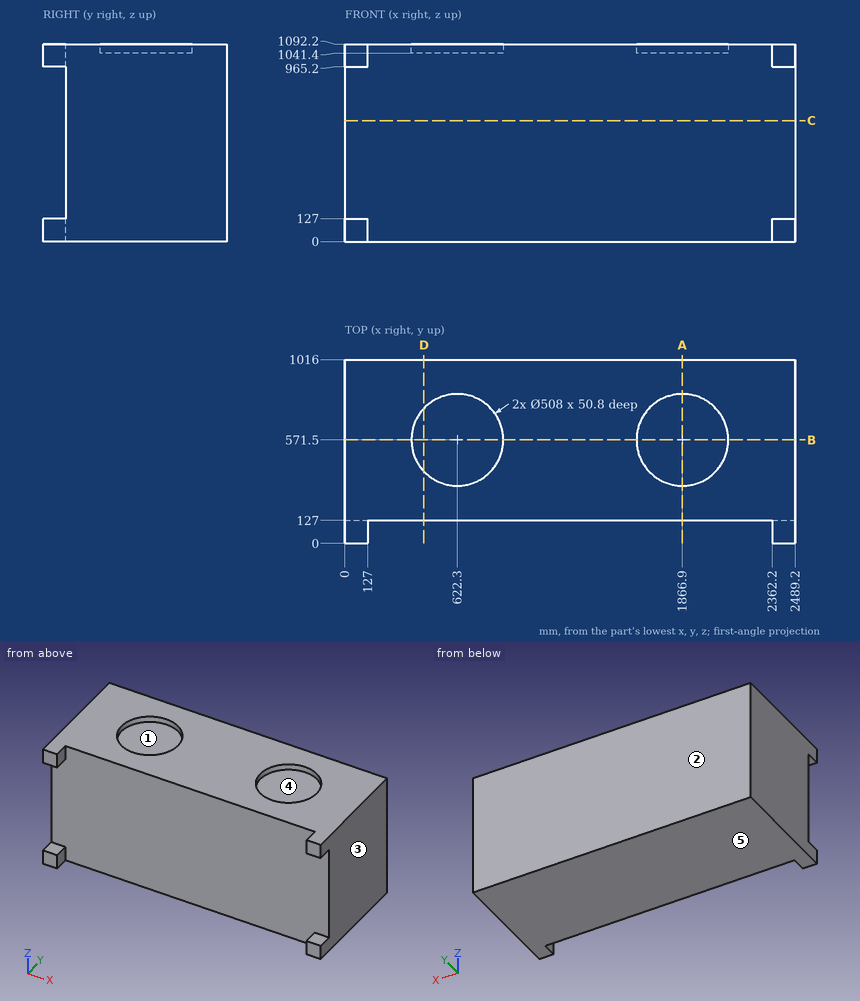
Design review of the part shown in the three views and the two pictorial views. Dimensions are in mm from the part's minimum x, y and z. A direction names the side the tool comes from. Round coordinates to 2 decimals unless told otherwise and drop trailing zeros. Order: outer loops, then holes, each group sorted by start corner. A loop starts at its lowest first (then second) coordinate and runs counter-clockwise, first axis right, second up.
(1) Take a section at B-B, the plane y = 571.5. State the section outline as (x, z) points, plus the area to 3 significant figures.
Working result:
outline: (0, 0) - (2489.2, 0) - (2489.2, 1092.2) - (2120.9, 1092.2) - (2120.9, 1041.4) - (1612.9, 1041.4) - (1612.9, 1092.2) - (876.3, 1092.2) - (876.3, 1041.4) - (368.3, 1041.4) - (368.3, 1092.2) - (0, 1092.2) - close
area: 2,670,000 mm2
(2) Take a section at C-C, the plane z = 668.5. State the section outline as (x, y) points, plus the area to 3 significant figures.
Working result:
outline: (0, 127) - (2489.2, 127) - (2489.2, 1016) - (0, 1016) - close
area: 2,210,000 mm2
(3) Take a section at A-A, the plane x = 1866.9. State the section outline as (y, z) points, plus the area to 3 significant figures.
Working result:
outline: (127, 0) - (1016, 0) - (1016, 1092.2) - (825.5, 1092.2) - (825.5, 1041.4) - (317.5, 1041.4) - (317.5, 1092.2) - (127, 1092.2) - close
area: 945,000 mm2
(4) For P1, Ø1, axis at x = 1114.5, z = 912.5, coming from the -Y side; P2, Ø3, axis at x = 1753.5, y = 791.5, coming from the +Z side, all flat-tipped, find the tip position at first contact; note any pin that passes through.
Working result:
P1: stops at y = 127
P2: stops at z = 1041.4
(5) Take a section at D-D, the plane x = 437.5. State the section outline as (y, z) points, plus the area to 3 significant figures.
Working result:
outline: (127, 0) - (1016, 0) - (1016, 1092.2) - (745.76, 1092.2) - (745.76, 1041.4) - (397.24, 1041.4) - (397.24, 1092.2) - (127, 1092.2) - close
area: 953,000 mm2
(6) Mouldability with a two-part tool opening along Y and no side actions: class the marked faces 1, 2 and 3 as released by +Y, released by -Y, zero draft, split by the parting line, or undercut.
Working result:
face 1: undercut
face 2: released by +Y
face 3: zero draft
(7) Wall thickness on L1, parallel to X at y = 571, z = 1060; L2, parallel to Y at x = 622, z = 1074; L3, parallel to Y at x = 2090.5, z = 662: over which ranges is each line inside the solid? List them lowest first.
Working result:
L1: x = 0 to 368.3, 876.3 to 1612.9, 2120.9 to 2489.2
L2: y = 127 to 317.5, 825.5 to 1016
L3: y = 127 to 1016
(8) Tool access review of the marked faces 4 and 5: name each direction out of +Z, -Z, +X, -X, +Y, -Y from which nothing blocks a thin tool from reaching the whole face with its end or side.
Working result:
face 4: +Z
face 5: -Z, +X, -X, +Y, -Y
